from build123d import *

# Parameters (mm, degrees)
ESBO_O2_R                  = 2.25
CORTE_EXTRUS_O2_DEPTH      = 19
ESBO_O7_R                  = 2.25
CORTE_EXTRUS_O6_DEPTH      = 3.329371528
CORTE_EXTRUS_O6_DEPTH_BACK = 20.716036402
CUT_EXTRUDE1_DEPTH         = 2.25
FILLET1_R                  = 0.5
CHAMFER1_SIZE              = 0.25
CHAMFER4_SIZE              = 0.25


with BuildPart() as part:
    # Esboço1 → Revolução1 (revolve)
    with BuildSketch(Plane.XY):
        Polygon((0, 33), (3, 33), (3, 13), (9, 13), (9, -13), (3, -13), (3, -17.5), (0, -17.5), (0, 0), align=None)
    revolve(axis=Axis((0, 0, 0), (0, 1, 0)))

    # Esboço2 → Corte-extrusão2 (cut, through all)
    with BuildSketch(Plane.ZY.offset(9)):
        Circle(ESBO_O2_R)
    extrude(amount=-CORTE_EXTRUS_O2_DEPTH, mode=Mode.SUBTRACT)

    # Esboço7 → Corte-extrusão6 (cut, two sides)
    with BuildSketch(Plane(origin=(-7.794228634, 0, 4.5), x_dir=(0.258819045, 0, 0.965925826), z_dir=(-0.965925826, 0, 0.258819045))) as corte_extrus_o6_sk:
        Circle(ESBO_O7_R)
    extrude(amount=CORTE_EXTRUS_O6_DEPTH, mode=Mode.SUBTRACT)
    extrude(corte_extrus_o6_sk.sketch, amount=-CORTE_EXTRUS_O6_DEPTH_BACK, mode=Mode.SUBTRACT)

    # Sketch1 → Cut-Extrude1 (cut, symmetric)
    with BuildSketch(Plane(origin=(0, 0, 0), x_dir=(1, 0, 0), z_dir=(0, 1, 0))):
        Polygon((9, 0), (-10.844388007, 0), (-10.42876147, -5.205920946), align=None)
    extrude(amount=CUT_EXTRUDE1_DEPTH, both=True, mode=Mode.SUBTRACT)

    # Fillet1
    fillet1_edges = [part.edges().sort_by_distance(p)[0] for p in [
        (-3, -13, 0),
        (-3, 13, 0),
    ]]
    fillet(fillet1_edges, radius=FILLET1_R)

    # Chamfer1
    chamfer1_edges = [part.edges().sort_by_distance(p)[0] for p in [
        (-3, -17.5, 0),
        (-3, 33, 0),
    ]]
    chamfer(chamfer1_edges, length=CHAMFER1_SIZE)

    # Chamfer4
    chamfer4_edges = [part.edges().sort_by_distance(p)[0] for p in [
        (-9, -13, 0),
        (-9, 13, 0),
    ]]
    chamfer(chamfer4_edges, length=CHAMFER4_SIZE)


solid = part.part
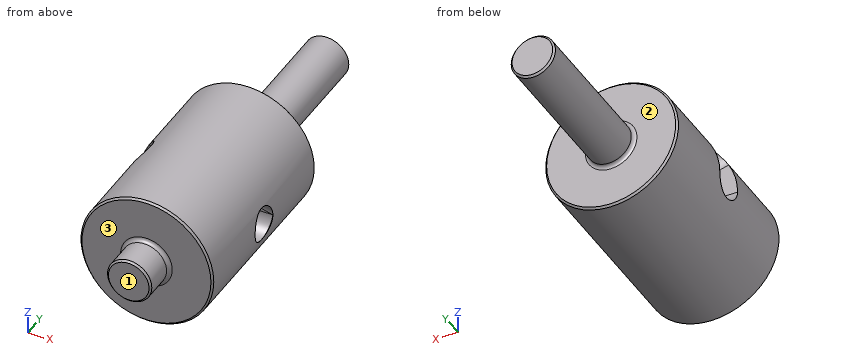
Design review of the part built by this model. Coordinates are the model's own, in mm. Face numbers are marked on the shaded views. A direction names the side the tool comes from. Coordinates: 2 decimals unless noted, no trailing zeros. Order: outer loops, then holes, each group sorted by start corner. A loop starts at its lowest first (then second) coordinate and runs counter-clockwise, first axis right, second up.
Item 1: Take a section at C-C, the plane y = 6.5. Write out the cut boundary in (x, z), then the cut area to 3 significant figures.
Item 2: For line 1 (Y direction, x = -3.5, z = 2.75); line 2 (Y direction, x = -4, z = 6.25); line 3 (Y direction, x = -1, z = 2), list the stretches that pass through material, from the lowest coordinate up.
Item 3: Take a section at B-B, the plane y = 22. Write out the cut boundary in (x, z).
Item 4: For pin 1 Ø5 at (x, z) = (-7, 0.5) entering from -Y; pin 2 Ø10 at (x, y) = (-5.5, -8) entering from -Z; pin 3 Ø5 at (x, y) = (-5.5, 12.5) entering from +Z, all flat-tipped, find the tip position at first contact; note any pin that passes through.
Item 5: For the marked faces 1, 2 and 3, list the 3-axis set-ups (+Z, -Z, +X, -X, +Y, -Y) from which the entire face can be reached by the end or side of a thin tool; tool diameter is ignored.
The answers:
1. outline: circle Ø18 at (0, 0)
1. area: 254 mm2
2. line 1: y = -13 to -2.25, 2.25 to 13
2. line 2: y = -13 to 13
2. line 3: y = -17.5 to -2.25, 2.25 to 33
3. outline: circle Ø6 at (0, 0)
4. pin 1: stops at y = -13
4. pin 2: stops at z = -8.99
4. pin 3: stops at z = 8.49
5. face 1: +Z, -Z, +X, -X, -Y
5. face 2: +Y
5. face 3: -Y
